Work out the finished part from the listing and answer in its coordinate system (mm). Face numbers are marked on the shaded views. A direction names the side the tool comes from. Coordinates: 2 decimals unless noted, no trailing zeros. Loops run counter-clockwise (first coordinate to the right, second up) from the corner with the lowest first, then second, coordinate; pieces in that order, holes last. Notation, with made-up numbers: (42.25, 49.5) - (67.25, 49.5) arc R19 cw to (67.25, 66.5) - close; hole circle Ø5 at (38, 36.5). An arc over 180 degrees is marked (long way). Write each question's results on one line, items separated by ' | '. Start each with the question number.
1. Find the intervals of material crossed by line 1 along Z through (x, y) = (30, 12); line 2 along Y through (x, z) = (36.5, -10) (3 decimals); line 3 along Y through (x, z) = (20, 1.25), in increasing order. Write a range as [from, to].
2. Determine the mould class of the marked faces 1, 2 and 3 for opening direction Y: released by +Y, released by -Y, zero draft, split by the parting line, or undercut.
3. Which of the six approach directions +Z, -Z, +X, -X, +Y, -Y give full straight-line access (tool end or side, diameter ignored) to the marked faces 4 and 5?
4. A cutting plane is placed at B-B on z = -20.5. State how many separate pieces and enclosed holes the cut face has, then the cut area to 3 significant figures.
5. Each of these flat-tipped pins is pushed along its axis until it touches: P1, Ø12, axis at y = 5.5, z = -31, coming from the -X side; P2, Ø3.5, axis at x = 38.9, y = 13.5, coming from the +Z side; P3, Ø3, axis at x = 26, z = -29, coming from the +Y side. Where does it stop, or does it pass through?
6. A cutting plane is placed at A-A on x = -1.5. Determine the outline of the cut face in (y, z) (3 decimals).
7. A cutting plane is placed at D-D on x = 8.5. Determine the outline of the cut face in (y, z) (3 decimals), then the cut area to 3 significant figures.
from build123d import *

# Parameters (mm, degrees)
BOSS_EXTRUDE1_START = 0.1
BOSS_EXTRUDE1_DEPTH = 3.2
BOSS_EXTRUDE4_DEPTH = 43
MIRROR9_START       = -12.580412483
MIRROR9_DEPTH       = 56.024226278
CUT_EXTRUDE1_START  = -41.930024
SKETCH5_W           = 10.7
SKETCH5_H           = 21.400046012
CUT_EXTRUDE1_DEPTH  = 41.930024


with BuildPart() as part:
    # Sketch1 → Boss-Extrude1 (new body)
    with BuildSketch(Plane.XY.offset(BOSS_EXTRUDE1_START)):
        with BuildLine():
            Line((6.5, -20.96501071), (40.371666845, -20.96501071))
            Line((40.371666845, -20.96501071), (46.843813692, -20.96501071))
            Line((46.843813692, -20.96501071), (46.843813692, -14.492829244))
            Line((46.843813692, -14.492829244), (46.843817152, 14.492909287))
            Line((46.843817152, 14.492909287), (46.843817152, 20.965012858))
            Line((46.843817152, 20.965012858), (40.371232335, 20.965012858))
            Line((40.371232335, 20.965012858), (-12.580412483, 20.965012858))
            Line((-12.580412483, 20.965012858), (-12.580412483, 14.9))
            Line((-12.580412483, 14.9), (6.5, 14.9))
            ThreePointArc((6.5, 14.9), (10.784081461, 13.885171119), (14.157668767, 11.056365661))
            Line((14.157668767, 11.056365661), (33.335287122, 11.056365661))
            add(Edge.make_bspline(
                [(33.335287122, 11.056365661), (33.738464028, 11.056365661), (34.553650563, 10.895055506), (35.583998517, 10.205191286), (36.273862737, 9.174843333), (36.435172892, 8.359656798), (36.435172892, 7.956479892)],
                knots=[-0.785360087, -0.785360087, -0.785360087, -0.785360087, -0.392680044, 0, 0.392680044, 0.785360087, 0.785360087, 0.785360087, 0.785360087], degree=3))
            Line((36.435172892, 7.956479892), (36.435172892, 7.38396472))
            ThreePointArc((36.435172892, 7.38396472), (39.928807231, 0), (36.435172892, -7.38396472))
            Line((36.435172892, -7.38396472), (36.435172892, -7.956479892))
            add(Edge.make_bspline(
                [(36.435172892, -7.956479892), (36.435172892, -8.359656798), (36.273862737, -9.174843333), (35.583998517, -10.205191286), (34.553650563, -10.895055506), (33.738464028, -11.056365661), (33.335287122, -11.056365661)],
                knots=[-0.785360087, -0.785360087, -0.785360087, -0.785360087, -0.392680044, 0, 0.392680044, 0.785360087, 0.785360087, 0.785360087, 0.785360087], degree=3))
            Line((33.335287122, -11.056365661), (14.157668767, -11.056365661))
            ThreePointArc((14.157668767, -11.056365661), (10.784081461, -13.885171119), (6.5, -14.9))
            Line((6.5, -14.9), (-12.580412483, -14.9))
            Line((-12.580412483, -14.9), (-12.580412483, -20.96501071))
            Line((-12.580412483, -20.96501071), (6.5, -20.96501071))
        make_face()
    extrude(amount=BOSS_EXTRUDE1_DEPTH)


with BuildPart() as body_2:
    # Mirror8: mirrored copy
    add(part.part.mirror(Plane.XY.offset(-19.8)))


with BuildPart() as part_1:
    add(part.part)

    add(body_2.part)  # Boss-Extrude4 merges body 2
    # Sketch3 → Boss-Extrude4 (add)
    with BuildSketch(Plane(origin=(0, 0, 0.1), x_dir=(-1, 0, 0), z_dir=(0, 0, -1))):
        with BuildLine():
            Line((-46.843817152, -20.96501071), (12.580412483, -20.96501071))
            Line((12.580412483, -20.96501071), (12.580412481, -17.56501071))
            Line((12.580412481, -17.56501071), (-40.344731515, -17.565009918))
            add(Edge.make_bspline(
                [(-40.344731515, -17.565009918), (-40.442934479, -17.56345098), (-40.546251638, -17.560214099), (-40.748160222, -17.540082036), (-40.848537497, -17.525369256), (-41.147208229, -17.466024859), (-41.34230873, -17.40685234), (-41.904876795, -17.173936033), (-42.248881792, -16.944079436), (-42.822875895, -16.370055351), (-43.052718695, -16.026081256), (-43.285678392, -15.463505278), (-43.344823049, -15.268405947), (-43.404196351, -14.969745759), (-43.418915361, -14.869354632), (-43.439033339, -14.667434906), (-43.442259272, -14.564125008), (-43.443813695, -14.465921992)],
                knots=[0, 0, 0, 0, 0.0625, 0.0625, 0.125, 0.125, 0.25, 0.25, 0.5, 0.5, 0.75, 0.75, 0.875, 0.875, 0.9375, 0.9375, 1, 1, 1, 1], degree=3))
            Line((-43.443813695, -14.465921992), (-43.443817149, 14.465924278))
            add(Edge.make_bspline(
                [(-43.443817149, 14.465924278), (-43.442258211, 14.564127242), (-43.43902133, 14.6674444), (-43.418889268, 14.869352985), (-43.404176488, 14.969730261), (-43.344832091, 15.268400993), (-43.285659572, 15.463501494), (-43.052743266, 16.026069561), (-42.822886669, 16.370074559), (-42.248862584, 16.944068663), (-41.904888488, 17.173911463), (-41.342312509, 17.406871161), (-41.147213178, 17.466015819), (-40.84855299, 17.52538912), (-40.748161863, 17.54010813), (-40.546242137, 17.560226109), (-40.442932239, 17.563452042), (-40.344729223, 17.565006465)],
                knots=[0, 0, 0, 0, 0.0625, 0.0625, 0.125, 0.125, 0.25, 0.25, 0.5, 0.5, 0.75, 0.75, 0.875, 0.875, 0.9375, 0.9375, 1, 1, 1, 1], degree=3))
            Line((-40.344729223, 17.565006465), (12.580412471, 17.565012858))
            Line((12.580412471, 17.565012858), (12.580412483, 20.965012858))
            Line((12.580412483, 20.965012858), (-46.843817152, 20.965012858))
            Line((-46.843817152, 20.965012858), (-46.843817152, -20.96501071))
        make_face()
    extrude(amount=BOSS_EXTRUDE4_DEPTH)


with BuildPart() as mirror9_tool:
    # Mirror9: read off the stored shape, not the designer's step
    # Mirror9 outline → Mirror9 (new body)
    with BuildSketch(Plane.YZ.offset(MIRROR9_START)):
        Polygon((17.541421356, -16.5), (16, -18.041421356), (16, -23.658578644), (16.641421356, -24.3), (17.565009661, -24.3), (17.565007122, -16.5), align=None)
        Polygon((-17.56501071, -24.3), (-16.641421356, -24.3), (-16, -23.658578644), (-16, -18.041421356), (-17.541421356, -16.5), (-17.56501071, -16.5), align=None)
    extrude(amount=MIRROR9_DEPTH)


with BuildPart() as part_2:
    add(part_1.part)


with BuildPart() as part_3:
    # Mirror9: joined with mirror9_tool
    add(part_2.part.fuse(mirror9_tool.part, tol=0.00001))

    # Sketch5 → Cut-Extrude1 (cut)
    with BuildSketch(Plane(origin=(0, 20.965012858, 0), x_dir=(1, 0, 0), z_dir=(0, 1, 0)).offset(CUT_EXTRUDE1_START)):
        with Locations((29.678807231, 20.899976994)):
            Rectangle(SKETCH5_W, SKETCH5_H)
    extrude(amount=CUT_EXTRUDE1_DEPTH, mode=Mode.SUBTRACT)

    # CSK for M2.5 Countersunk Flat Head Screw1: read off the stored shape, not the designer's step
    # CSK for M2.5 Countersunk Flat Head S 2 → CSK for M2.5 Countersunk Flat Head Screw1 (revolve, cut)
    with BuildSketch(Plane(origin=(20, -14, 0), x_dir=(1, 0, 0), z_dir=(0, -1, 0))):
        Polygon((1.45, -41.6), (1.45, -39.7), (0, -39.7), (0, -42.9), (2.75, -42.9), align=None)
        Polygon((0, 0.1), (1.45, 0.1), (1.45, 2), (2.75, 3.3), (0, 3.3), align=None)
    revolve(axis=Axis((20, -14, 0), (0, 0, 1)), mode=Mode.SUBTRACT)

    # CSK for M2.5 Countersunk Flat Head S 3 o → CSK for M2.5 Countersunk Flat Head S 3 (revolve, cut)
    with BuildSketch(Plane(origin=(20, 14, 0), x_dir=(1, 0, 0), z_dir=(0, -1, 0))):
        Polygon((1.45, -41.6), (1.45, -39.7), (0, -39.7), (0, -42.9), (2.75, -42.9), align=None)
        Polygon((0, 0.1), (1.45, 0.1), (1.45, 2), (2.75, 3.3), (0, 3.3), align=None)
    revolve(axis=Axis((20, 14, 0), (0, 0, 1)), mode=Mode.SUBTRACT)

    # CSK for M2.5 Countersunk Flat Head S 4 o → CSK for M2.5 Countersunk Flat Head S 4 (revolve, cut)
    with BuildSketch(Plane(origin=(38.9, 13.5, 0), x_dir=(1, 0, 0), z_dir=(0, -1, 0))):
        Polygon((1.45, -41.6), (1.45, -39.7), (0, -39.7), (0, -42.9), (2.75, -42.9), align=None)
        Polygon((0, 0.1), (1.45, 0.1), (1.45, 2), (2.75, 3.3), (0, 3.3), align=None)
    revolve(axis=Axis((38.9, 13.5, 0), (0, 0, 1)), mode=Mode.SUBTRACT)

    # CSK for M2.5 Countersunk Flat Head S 5 o → CSK for M2.5 Countersunk Flat Head S 5 (revolve, cut)
    with BuildSketch(Plane(origin=(38.9, -13.5, 0), x_dir=(1, 0, 0), z_dir=(0, -1, 0))):
        Polygon((1.45, -41.6), (1.45, -39.7), (0, -39.7), (0, -42.9), (2.75, -42.9), align=None)
        Polygon((0, 0.1), (1.45, 0.1), (1.45, 2), (2.75, 3.3), (0, 3.3), align=None)
    revolve(axis=Axis((38.9, -13.5, 0), (0, 0, 1)), mode=Mode.SUBTRACT)


solid = part_3.part
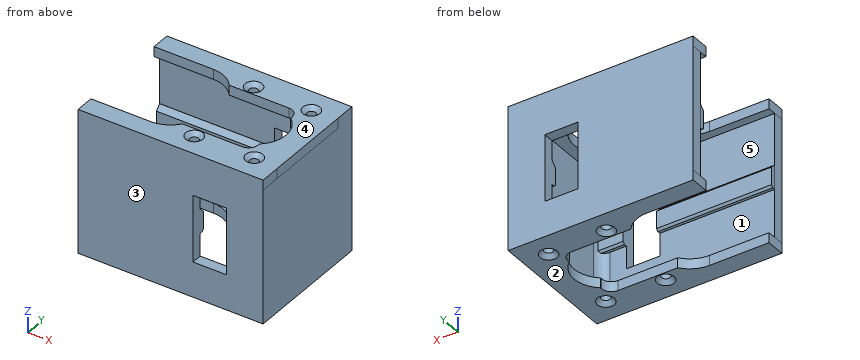
Values:
1) line 1: [-42.9, -39.7], [0.1, 3.3] | line 2: [-20.965, -17.565], [17.565, 20.965] | line 3: [-20.97, -15.45], [-12.55, -11.06], [11.06, 12.55], [15.45, 20.97]
2) face 1: undercut | face 2: zero draft | face 3: released by -Y
3) face 4: +Z, +X, -X, +Y, -Y | face 5: -X
4) separate pieces: 3 | enclosed holes: 0 | area: 593 mm^2
5) P1: x = 43.44 | P2: z = 2.3 | P3: through
6) outline: (-20.965, -42.9) - (-14.9, -42.9) - (-14.9, -39.7) - (-17.565, -39.7) - (-17.565, -24.3) - (-16.641, -24.3) - (-16, -23.659) - (-16, -18.041) - (-17.541, -16.5) - (-17.565, -16.5) - (-17.565, 0.1) - (-14.9, 0.1) - (-14.9, 3.3) - (-20.965, 3.3) - close; (14.9, -42.9) - (20.965, -42.9) - (20.965, 3.3) - (14.9, 3.3) - (14.9, 0.1) - (17.565, 0.1) - (17.565, -16.5) - (17.541, -16.5) - (16, -18.041) - (16, -23.659) - (16.641, -24.3) - (17.565, -24.3) - (17.565, -39.7) - (14.9, -39.7) - close
7) outline: (-20.965, -42.9) - (-14.688, -42.9) - (-14.688, -39.7) - (-17.565, -39.7) - (-17.565, -24.3) - (-16.641, -24.3) - (-16, -23.659) - (-16, -18.041) - (-17.541, -16.5) - (-17.565, -16.5) - (-17.565, 0.1) - (-14.688, 0.1) - (-14.688, 3.3) - (-20.965, 3.3) - close; (14.688, -42.9) - (20.965, -42.9) - (20.965, 3.3) - (14.688, 3.3) - (14.688, 0.1) - (17.565, 0.1) - (17.565, -16.5) - (17.541, -16.5) - (16, -18.041) - (16, -23.659) - (16.641, -24.3) - (17.565, -24.3) - (17.565, -39.7) - (14.688, -39.7) - close | area: 373 mm^2
